from build123d import *

# Parameters (mm, degrees)
SKETCH_2_R          = 1.55
SKETCH_2_R_2        = 1.25
SKETCH_2_R_3        = 1.75
SKETCH_2_R_4        = 2.55
EXTRUDE_1_DEPTH     = 4
FILLET_1_R          = 20
SKETCH_4_R          = 12.5
CUT_EXTRUDE_3_DEPTH = 4
EXTRUDE_START       = -4
EXTRUDE_2_DEPTH     = 4
FILLET_5_R          = 5
SKETCH_10_R         = 2.55
CUT_EXTRUDE_6_DEPTH = 10
EXTRUDE_3_DEPTH     = 4
FILLET_6_R          = 5
SKETCH_12_R         = 2.55
CUT_EXTRUDE_7_DEPTH = 4
CUT_EXTRUDE_8_DEPTH = 4
FILLET_7_R          = 3


with BuildPart() as part:
    # 草图2 → 凸台-拉伸1 (new body)
    with BuildSketch(Plane.XY.offset(50)):
        with BuildLine():
            Line((-25.35656347, 96.806195191), (-36.91814256, 90.799541468))
            ThreePointArc((-36.91814256, 90.799541468), (-37.739334229, 90.232640986), (-38.394655297, 89.480121078))
            Line((-38.394655297, 89.480121078), (-45.6586136, 78.66416482))
            ThreePointArc((-45.6586136, 78.66416482), (-52.612848944, 64.027729908), (-55, 48))
            Line((-55, 48), (-55, 10))
            ThreePointArc((-55, 10), (-53.535533906, 6.464466094), (-50, 5))
            Line((-50, 5), (-34.292856399, 5))
            ThreePointArc((-34.292856399, 5), (0, -7), (34.292856399, 5))
            Line((34.292856399, 5), (50, 5))
            ThreePointArc((50, 5), (53.535533906, 6.464466094), (55, 10))
            Line((55, 10), (55, 48))
            ThreePointArc((55, 48), (52.612848944, 64.027729908), (45.6586136, 78.66416482))
            Line((45.6586136, 78.66416482), (38.394655297, 89.480121078))
            ThreePointArc((38.394655297, 89.480121078), (37.739334229, 90.232640986), (36.91814256, 90.799541468))
            Line((36.91814256, 90.799541468), (25.35656347, 96.806195191))
            ThreePointArc((25.35656347, 96.806195191), (0, 103), (-25.35656347, 96.806195191))
        make_face()
        with Locations((-35.074028853, 87.25)):
            Circle(SKETCH_2_R, mode=Mode.SUBTRACT)
        with Locations((-18, 72)):
            Circle(SKETCH_2_R_2, mode=Mode.SUBTRACT)
        with Locations((-12.07, 61)):
            Circle(SKETCH_2_R_3, mode=Mode.SUBTRACT)
        with Locations((-12.07, 35)):
            Circle(SKETCH_2_R_3, mode=Mode.SUBTRACT)
        with Locations((-18, 24)):
            Circle(SKETCH_2_R_2, mode=Mode.SUBTRACT)
        with Locations((18, 72)):
            Circle(SKETCH_2_R_2, mode=Mode.SUBTRACT)
        with Locations((12.07, 61)):
            Circle(SKETCH_2_R_3, mode=Mode.SUBTRACT)
        with Locations((12.07, 35)):
            Circle(SKETCH_2_R_3, mode=Mode.SUBTRACT)
        with Locations((35.074028853, 87.25)):
            Circle(SKETCH_2_R, mode=Mode.SUBTRACT)
        with Locations((18, 24)):
            Circle(SKETCH_2_R_2, mode=Mode.SUBTRACT)
        with Locations((-50, 10)):
            Circle(SKETCH_2_R_4, mode=Mode.SUBTRACT)
        with Locations((50, 10)):
            Circle(SKETCH_2_R_4, mode=Mode.SUBTRACT)
    extrude(amount=EXTRUDE_1_DEPTH)

    # 圆角1
    fillet_1_edges = [part.edges().sort_by_distance(p)[0] for p in [
        (-34.292856399, 5, 52),
        (34.292856399, 5, 52),
    ]]
    fillet(fillet_1_edges, radius=FILLET_1_R)

    # 草图4 → 切除-拉伸3 (cut)
    with BuildSketch(Plane.XY.offset(54)):
        with Locations((0, 48)):
            Circle(SKETCH_4_R)
    extrude(amount=-CUT_EXTRUDE_3_DEPTH, mode=Mode.SUBTRACT)

    # 草图8 → 凸台-拉伸2 (add)
    with BuildSketch(Plane.XY.offset(54).offset(EXTRUDE_START)):
        with BuildLine():
            Line((-55, 103), (-55, 48))
            ThreePointArc((-55, 48), (-52.612848944, 64.027729908), (-45.6586136, 78.66416482))
            Line((-45.6586136, 78.66416482), (-38.394655297, 89.480121078))
            ThreePointArc((-38.394655297, 89.480121078), (-37.739334229, 90.232640986), (-36.91814256, 90.799541468))
            Line((-36.91814256, 90.799541468), (-25.35656347, 96.806195191))
            ThreePointArc((-25.35656347, 96.806195191), (-13.051039509, 101.429115356), (0, 103))
            Line((0, 103), (-55, 103))
        make_face()
    extrude_2 = extrude(amount=EXTRUDE_2_DEPTH)

    # 镜向4: 凸台-拉伸2 across plane
    add(extrude_2.mirror(Plane(origin=(0, 0, 0), x_dir=(0, 0, 1), z_dir=(1, 0, 0))))

    # 圆角5
    fillet_5_edges = [part.edges().sort_by_distance(p)[0] for p in [
        (-55, 103, 52),
        (55, 103, 52),
    ]]
    fillet(fillet_5_edges, radius=FILLET_5_R)

    # 草图10 → 切除-拉伸6 (cut)
    with BuildSketch(Plane.XY.offset(54)):
        with Locations((-50, 98)):
            Circle(SKETCH_10_R)
        with Locations((50, 98)):
            Circle(SKETCH_10_R)
    extrude(amount=-CUT_EXTRUDE_6_DEPTH, mode=Mode.SUBTRACT)

    # 草图11 → 凸台-拉伸3 (add)
    with BuildSketch(Plane(origin=(0, 0, 50), x_dir=(-1, 0, 0), z_dir=(0, 0, -1))):
        with BuildLine():
            ThreePointArc((-50, 5), (-53.535533906, 6.464466094), (-55, 10))
            Line((-55, 10), (-55, -7))
            Line((-55, -7), (0, -7))
            ThreePointArc((0, -7), (-15.556349186, -4.754146756), (-29.842251926, 1.8))
            ThreePointArc((-29.842251926, 1.8), (-35.037125649, 4.183326093), (-40.693979899, 5))
            Line((-40.693979899, 5), (-50, 5))
        make_face()
        with BuildLine():
            ThreePointArc((29.842251926, 1.8), (15.556349186, -4.754146756), (0, -7))
            Line((0, -7), (55, -7))
            Line((55, -7), (55, 10))
            ThreePointArc((55, 10), (53.535533906, 6.464466094), (50, 5))
            Line((50, 5), (40.693979899, 5))
            ThreePointArc((40.693979899, 5), (35.037125649, 4.183326093), (29.842251926, 1.8))
        make_face()
    extrude(amount=-EXTRUDE_3_DEPTH)

    # 圆角6
    fillet_6_edges = [part.edges().sort_by_distance(p)[0] for p in [
        (55, -7, 52),
        (-55, -7, 52),
    ]]
    fillet(fillet_6_edges, radius=FILLET_6_R)

    # 草图12 → 切除-拉伸7 (cut)
    with BuildSketch(Plane(origin=(0, 0, 50), x_dir=(-1, 0, 0), z_dir=(0, 0, -1))):
        with Locations((-50, -2)):
            Circle(SKETCH_12_R)
        with Locations((50, -2)):
            Circle(SKETCH_12_R)
    extrude(amount=-CUT_EXTRUDE_7_DEPTH, mode=Mode.SUBTRACT)

    # 草图13 → 切除-拉伸8 (cut)
    with BuildSketch(Plane.XY.offset(54)):
        with BuildLine():
            Line((-23.852223166, 66.195368917), (-45, 87.343145751))
            Line((-45, 87.343145751), (-45, 18.82410191))
            Line((-45, 18.82410191), (-26.091936894, 33.19422987))
            ThreePointArc((-26.091936894, 33.19422987), (-29.931147249, 50.031360229), (-23.852223166, 66.195368917))
        make_face()
        with BuildLine():
            Line((0, 70.5), (0, 93))
            Line((0, 93), (-30.514718626, 93))
            Line((-30.514718626, 93), (-6.923133414, 69.408414788))
            ThreePointArc((-6.923133414, 69.408414788), (-3.504330697, 70.225428373), (0, 70.5))
        make_face()
        with BuildLine():
            Line((0, 3), (0, 25.5))
            ThreePointArc((0, 25.5), (-3.504330697, 25.774571627), (-6.923133414, 26.591585212))
            Line((-6.923133414, 26.591585212), (-30.514718626, 3))
            Line((-30.514718626, 3), (0, 3))
        make_face()
    cut_extrude_8 = extrude(amount=-CUT_EXTRUDE_8_DEPTH, mode=Mode.SUBTRACT)

    # 镜向5: 切除-拉伸8 across plane
    add(cut_extrude_8.mirror(Plane(origin=(0, 0, 0), x_dir=(0, 0, 1), z_dir=(1, 0, 0))), mode=Mode.SUBTRACT)

    # 圆角7
    fillet_7_edges = [part.edges().sort_by_distance(p)[0] for p in [
        (-30.514718626, 3, 52),
        (-6.923133414, 26.591585212, 52),
        (-6.923133414, 69.408414788, 52),
        (-30.514718626, 93, 52),
        (-23.852223166, 66.195368917, 52),
        (-26.091936894, 33.19422987, 52),
        (-45, 18.82410191, 52),
        (-45, 87.343145751, 52),
        (6.923133414, 26.591585212, 52),
        (30.514718626, 3, 52),
        (30.514718626, 93, 52),
        (6.923133414, 69.408414788, 52),
        (26.091936894, 33.19422987, 52),
        (23.852223166, 66.195368917, 52),
        (45, 87.343145751, 52),
        (45, 18.82410191, 52),
    ]]
    fillet(fillet_7_edges, radius=FILLET_7_R)


solid = part.part
Read the model definition and answer for the solid it produces. Units are mm, in the model's axes. A direction names the side the tool comes from. Give positions to 0.01 mm unless a question says otherwise; leave off trailing zeros. Loops run counter-clockwise (first coordinate to the right, second up) from the corner with the lowest first, then second, coordinate; pieces in that order, holes last. Notation, with made-up numbers: (16, 71.5) -> (22, 71.5) arc R18 ccw to (22, 95.5) -> close; hole circle Ø4 at (71.25, -31). An arc over 180 degrees is marked (long way). Answer as CSV lines item,"result".
Item 1: Find section D-D on z = 51.55. State how many separate pieces and enclosed holes the cut face has, plus the area to 3 significant figures.
Returned:
separate pieces,"1"
enclosed holes,"21"
area,"7,920 mm²"
Item 2: Find section A-A on y = 48. Give the vertices of the cut face in (x, z), plus the area to 3 significant figures.
Returned:
outline,"(-55, 50) -> (-45, 50) -> (-45, 54) -> (-55, 54) -> close; (-30, 50) -> (-12.5, 50) -> (-12.5, 54) -> (-30, 54) -> close; (12.5, 50) -> (30, 50) -> (30, 54) -> (12.5, 54) -> close; (45, 50) -> (55, 50) -> (55, 54) -> (45, 54) -> close"
area,"220 mm²"
Item 3: Find section B-B on x = -18. Give the vertices of the cut face in (y, z).
Returned:
outline,"(-7, 50) -> (3, 50) -> (3, 54) -> (-7, 54) -> close; (15.51, 50) -> (22.75, 50) -> (22.75, 54) -> (15.51, 54) -> close; (25.25, 50) -> (70.75, 50) -> (70.75, 54) -> (25.25, 54) -> close; (73.25, 50) -> (80.49, 50) -> (80.49, 54) -> (73.25, 54) -> close; (93, 50) -> (103, 50) -> (103, 54) -> (93, 54) -> close"
Item 4: For faces 5 (the face through (43.194, 82.853, 51.972)), 6 (the face through (-54, -5, 52)), determine the directions among +Z, -Z, +X, -X, +Y, -Y from which every point of the face is accessible in a straight line to the end or side of a thin tool.
Returned:
face 5,"+Z, -Z"
face 6,"+Z, -Z, -X, -Y"
Item 5: Consider line 1 (Y direction, x = 50, z = 52.65); line 2 (X direction, y = 87.25, z = 51.8); line 3 (X direction, y = 47.5, z = 50.6). Determine where each line is inside the solid, lowest interval first. Write a range as [from, to].
Returned:
line 1,"y = [-7, -4.55], [0.55, 7.45], [12.55, 95.45], [100.55, 103]"
line 2,"x = [-55, -36.62], [-33.52, -24.76], [24.76, 33.52], [36.62, 55]"
line 3,"x = [-55, -45], [-30, -12.49], [12.49, 30], [45, 55]"
Item 6: Find section C-C on y = 10. Give the vertices of the cut face in (x, z).
Returned:
outline,"(-55, 50) -> (-52.55, 50) -> (-52.55, 54) -> (-55, 54) -> close; (-47.45, 50) -> (-23.51, 50) -> (-23.51, 54) -> (-47.45, 54) -> close; (23.51, 50) -> (47.45, 50) -> (47.45, 54) -> (23.51, 54) -> close; (52.55, 50) -> (55, 50) -> (55, 54) -> (52.55, 54) -> close"
Item 7: Determine the mould class of faces 1 (the face through (55, 49, 52)), 2 (the face through (-26.024, 91.194, 51.972)), 3 (the face through (17.84, 73.24, 51.97)), 4 (the face through (1, 61, 54)) for opening direction X: +X half, -X half, draft (parallel to the pull), parting line (faces both ways), or undercut.
Returned:
face 1,"+X half"
face 2,"undercut"
face 3,"undercut"
face 4,"draft"
Item 8: Each of these flat-tipped pins is pushed along its axis until it touches: pin 1 (4.5 mm diameter, centred on x = 50, y = -2, fed in from +Z); pin 2 (5 mm diameter, centred on x = -35.07, y = 87.25, fed in from +Z). Where does it stop, or does it pass through?
Returned:
pin 1,"passes through"
pin 2,"stops at z = 54"
